Design review of the part built by this model. Coordinates are the model's own, in mm. A direction names the side the tool comes from. Coordinates: 2 decimals unless noted, no trailing zeros. Loops run counter-clockwise (first coordinate to the right, second up) from the corner with the lowest first, then second, coordinate; pieces in that order, holes last. Notation, with made-up numbers: M 10,56 L 56,56 A30 ccw 56,80 Z; hole C 24,59 d9. An arc over 180 degrees is marked long. Answer as a JSON object with one key per item and string values. Group by question number.
1. Consider section B-B (z = 78.5). State the section outline as (x, y) points, then the cut area to 3 significant figures.
2. Consider section D-D (z = 56). State the section outline as (x, y) points, then the cut area to 3 significant figures.
3. Insertion check: pin 1 (6 mm diameter, centred on y = -1, z = 45, fed in from -X); pin 2 (4 mm diameter, centred on y = -1, z = 48, fed in from -X); pin 3 (5 mm diameter, centred on x = 15, z = 15.5, fed in from +Y). Each pin has a flat end and moves straight along its axis. Give the tip position at first contact, or say it passes through.
4. To check wall thickness, follow probe 1 along Z at (x, y) = (17.5, -16.5); probe 2 along X at (y, z) = (-10.5, 56); probe 3 along Y at (x, z) = (3.5, 51.5). State the ranges of each line that lie inside material, in increasing order.
5. Consider section C-C (z = 13.5). State the section outline as (x, y) points, then the cut area to 3 significant figures.
6. Consider section A-A (x = 0). State the section outline as (y, z) points, then the cut area to 3 significant figures.
7. Machinability: for faces 1 (the flat face through (23.4, 3.8, 60)), 2 (the flat face through (21.752, 12.325, 72.325)), which of the approach directions +Z, -Z, +X, -X, +Y, -Y give a long, thin tool a straight path to every point of the face, cutting with its end or side? Answer none if there is none.
from build123d import *

# Parameters (mm, degrees)
F3_DEPTH = 25


with BuildPart() as f1:
    # F0 (on Front) → F1 (revolve)
    with BuildSketch(Plane.XZ):
        Polygon((-18.250227, 0), (0, 0), (0, 60), (-23.499547, 60), align=None)
    revolve(axis=Axis((0, 0, 72.624769), (0, 0, 1)))

    # F2 (on face) → F3 (join)
    with BuildSketch(Plane.XY.offset(60)):
        Polygon((-14.433757, 25), (-28.867513, 0), (-14.433757, -25), (14.433757, -25), (28.867513, 0), (14.433757, 25), align=None)
    extrude(amount=F3_DEPTH)


solid = f1.part
Findings below:
{
 "1": {"outline": "M -28.87,0 L -14.43,-25 L 14.43,-25 L 28.87,0 L 14.43,25 L -14.43,25 Z", "area": "2,170 mm^2"},
 "2": {"outline": "C 0,0 d46.3", "area": "1,680 mm^2"},
 "3": {"pin 1": "stops at x = -22.44", "pin 2": "stops at x = -22.61", "pin 3": "stops at y = 15.12"},
 "4": {"probe 1": "z = 60 to 85", "probe 2": "x = -20.63 to 20.63", "probe 3": "y = -22.49 to 22.49"},
 "5": {"outline": "C 0,0 d38.86", "area": "1,190 mm^2"},
 "6": {"outline": "M -25,60 L -23.5,60 L -18.25,0 L 18.25,0 L 23.5,60 L 25,60 L 25,85 L -25,85 Z", "area": "3,750 mm^2"},
 "7": {"face 1": "-Z", "face 2": "+Z, -Z, +X, +Y"}
}
